Read the model definition and answer for the solid it produces. Units are mm, in the model's axes. Face numbers are marked on the shaded views. A direction names the side the tool comes from. Coordinates: 2 decimals unless noted, no trailing zeros. Loops run counter-clockwise (first coordinate to the right, second up) from the corner with the lowest first, then second, coordinate; pieces in that order, holes last. Notation, with made-up numbers: (-34, -1) -> (-4, -1) arc R6 cw to (-4, 8) -> close; hole circle Ø1 at (78, 44). An arc over 180 degrees is marked (long way). Answer as a JSON object with one key per item and string values. Group by question number.
1) Section A-A, the plane z = 70 is taken. Give the vertices of the cut face in (x, y), plus the area to 3 significant figures.
2) Section B-B, the plane y = 34.5 is taken. Give the vertices of the cut face in (x, z).
3) Consider probe 1 along Y at (x, z) = (-14, 35.5); probe 2 along X at (y, z) = (32, 58.5); probe 3 along X at (y, z) = (30, 39). Determine where each line is inside the solid, lowest interval first. Write a range as [from, to].
4) Determine the mould class of the marked faces 1, 2 and 3 for opening direction Y: released by +Y, released by -Y, zero draft, split by the parting line, or undercut.
5) Section C-C, the plane x = -21 is taken. Give the vertices of the cut face in (y, z).
6) Which of the six approach directions +Z, -Z, +X, -X, +Y, -Y give full straight-line access (tool end or side, diameter ignored) to the marked faces 4 and 5?
from build123d import *

# Parameters (mm, degrees)
F0_W     = 76.2
F0_H     = 76.2
F1_DEPTH = 76.2
F3_DEPTH = 76.2


with BuildPart() as f1:
    # F0 (on Top) → F1 (new body)
    with BuildSketch(Plane.XY):
        with Locations((-7.110626, 25.808547)):
            Rectangle(F0_W, F0_H)
    extrude(amount=F1_DEPTH)

    # F2 (on face) → F3 (cut)
    with BuildSketch(Plane.XY.offset(76.2)):
        Polygon((-8.220765, 10.149787), (7.438689, 19.913918), (2.991485, 37.824227), (-15.416492, 39.129274), (-22.346044, 22.02553), align=None)
    extrude(amount=-F3_DEPTH, mode=Mode.SUBTRACT)


solid = f1.part
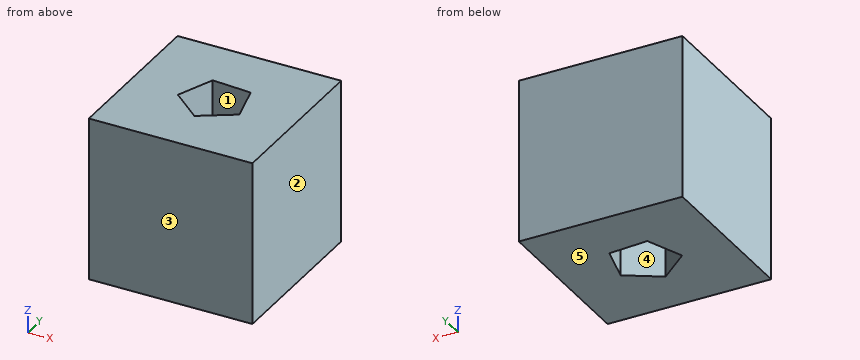
Determined:
{
 "1": {"outline": "(-45.21, -12.29) -> (30.99, -12.29) -> (30.99, 63.91) -> (-45.21, 63.91) -> close; hole (-22.35, 22.03) -> (-8.22, 10.15) -> (7.44, 19.91) -> (2.99, 37.82) -> (-15.42, 39.13) -> close", "area": "5,220 mm²"},
 "2": {"outline": "(-45.21, 0) -> (-17.29, 0) -> (-17.29, 76.2) -> (-45.21, 76.2) -> close; (3.82, 0) -> (30.99, 0) -> (30.99, 76.2) -> (3.82, 76.2) -> close"},
 "3": {"probe 1": "[-12.29, 15.01], [39.03, 63.91]", "probe 2": "[-45.21, -18.3], [4.44, 30.99]", "probe 3": "[-45.21, -19.12], [4.93, 30.99]"},
 "4": {"face 1": "undercut", "face 2": "zero draft", "face 3": "released by -Y"},
 "5": {"outline": "(-12.29, 0) -> (20.89, 0) -> (20.89, 76.2) -> (-12.29, 76.2) -> close; (25.35, 0) -> (63.91, 0) -> (63.91, 76.2) -> (25.35, 76.2) -> close"},
 "6": {"face 4": "+Z, -Z", "face 5": "-Z, +X, -X, +Y, -Y"}
}
